Could you check a few things on this model? Use its own coordinates, in mm. A direction names the side the tool comes from. Coordinates: 2 decimals unless noted, no trailing zeros. Order: outer loops, then holes, each group sorted by start corner. A loop starts at its lowest first (then second) coordinate and runs counter-clockwise, first axis right, second up. Notation, with made-up numbers: (37, 35.25) - (46, 35.25) arc R21 ccw to (46, 58.25) - close; hole circle Ø7 at (19.5, 61.5). An arc over 180 degrees is marked (long way). One line per item, written item: value. Start each with the question number.
from build123d import *

# Parameters (mm, degrees)
F1_DEPTH = 20


with BuildPart() as f1:
    # F0 (on Front) → F1 (new body, symmetric)
    with BuildSketch(Plane.XZ):
        with BuildLine():
            Line((-211.000333, 279.24695), (-211.000333, 349.999326))
            Line((-211.000333, 349.999326), (-215.000333, 349.999326))
            Line((-215.000333, 349.999326), (-215.000333, 281.230967))
            ThreePointArc((-215.000333, 281.230967), (0.004068, -354), (214.993869, 281.235908))
            Line((214.993869, 281.235908), (214.999667, 349.999663))
            Line((214.999667, 349.999663), (210.999667, 350))
            Line((210.999667, 350), (210.993702, 279.251961))
            ThreePointArc((210.993702, 279.251961), (0.004156, -350), (-211.000333, 279.24695))
        make_face()
    extrude(amount=F1_DEPTH, both=True)


solid = f1.part
Q1. I want a section at C-C on y = 14. Please give me the cut outline in (x, z).
Q2. If I drill on L1, parallel to X at y = -9, z = 0; L2, parallel to X at y = 0, z = 105.5; L3, parallel to Z at x = -319, y = 12.5, over which ranges is the centre line in solid material (lowest first)?
Q3. We'd pull the mould along X, two halves only. Please class faces 1 (the flat face through (-343, -20, 78)), 2 (the cylindrical face through (12.225, -0.28, -349.786)), 3 (the flat face through (-215, 0, 316)): +X half, -X half, draft (parallel to the pull), parting line (faces both ways), or undercut.
Q4. I want a section at B-B on x = 304. Please give me the cut outline in (y, z).
Q5. Which directions (+Z, -Z, +X, -X, +Y, -Y) give clear straight access to the entire face, cutting with the end or side of a thin tool? Please do faces 4 (the flat face through (-211, 0, 314)), 5 (the cylindrical face through (-12.328, -0.28, -353.785)).
Q6. I'm going to push flat-ended pins straight in: pin 1 (1.5 mm diameter, centred on y = -4.5, z = -269, fed in from +X); pin 2 (1 mm diameter, centred on x = 137.5, y = 14, fed in from +Z); pin 3 (1 mm diameter, centred on x = 98.5, y = 0, fed in from +Z). Where does each tip first touch, or does it pass through?
Values follow:
1. outline: (-215, 281.23) arc R354 ccw (long way) to (214.99, 281.24) - (215, 350) - (211, 350) - (210.99, 279.25) arc R350 cw (long way) to (-211, 279.25) - (-211, 350) - (-215, 350) - close
2. L1: x = -354 to -350, 350 to 354
2. L2: x = -337.91 to -333.72, 333.72 to 337.91
2. L3: z = -153.48 to -144.01, 144.01 to 153.48
3. face 1: draft
3. face 2: undercut
3. face 3: -X half
4. outline: (-20, -181.38) - (20, -181.38) - (20, -173.45) - (-20, -173.45) - close; (-20, 173.45) - (20, 173.45) - (20, 181.38) - (-20, 181.38) - close
5. face 4: +Z, +Y, -Y
5. face 5: +Y, -Y
6. pin 1: stops at x = 230.99
6. pin 2: stops at z = -321.65
6. pin 3: stops at z = -335.71
